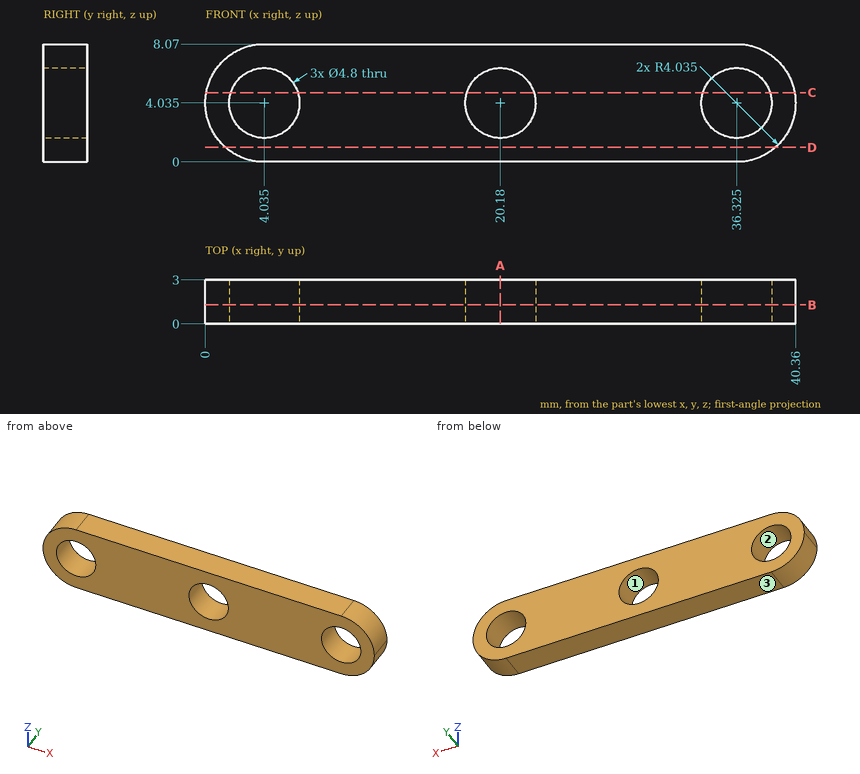
Verification items for this drawing (mm, ordinates from the low corner). Give positions to 0.01 mm unless a question says otherwise; leave off trailing zeros. Write each loop counter-clockwise with the first axis right and the second up, starting at its lowest first coordinate (ties: lowest second). Pieces come first, ordered by that corner, then holes. Notation, with made-up numbers: (66.5, 59) -> (70.5, 59) arc R16 ccw to (70.5, 77) -> close; hole circle Ø6 at (-2, 1). An arc over 180 degrees is marked (long way). Use one line per item in the form item = value.
Item 1: Depth check by flat-ended pin: pin 1 Ø1.5 at (x, z) = (24, 2.5) entering from -Y. Enter the tip coordinate at first touch or a pass-through.
Results list:
pin_1 = 0
Item 2: Scan lines: line 1 (X direction, y = 1.3, z = 4.25); line 2 (X direction, y = 1.5, z = 4.75); line 3 (Z direction, x = 18, y = 1.55). Record each from-to range of solid material in increasing order.
Results list:
line_1 = 0.01 to 1.64, 6.43 to 17.79, 22.57 to 33.93, 38.72 to 40.35
line_2 = 0.06 to 1.74, 6.33 to 17.89, 22.47 to 34.03, 38.62 to 40.3
line_3 = 0 to 3.03, 5.04 to 8.07
Item 3: Sectioned sample at D-D on z = 1. Enter the section's corners in (x, y).
Results list:
outline = (1.38, 0) -> (38.98, 0) -> (38.98, 3) -> (1.38, 3) -> close
Item 4: Mould release check, pull along X, two halves, no side actions. Record for the marked faces 1, 2 and 3: released by +X, released by -X, zero draft, split by the parting line, or undercut.
Results list:
face_1 = undercut
face_2 = undercut
face_3 = zero draft
Item 5: Sectioned sample at B-B on y = 1.3. Enter the section's corners in (x, z) (3 decimals).
Results list:
outline = (4.035, 0) -> (36.325, 0) arc R4.035 ccw to (36.325, 8.07) -> (4.035, 8.07) arc R4.035 ccw to start; hole circle Ø4.8 at (4.035, 4.035); hole circle Ø4.8 at (20.18, 4.035); hole circle Ø4.8 at (36.325, 4.035)
Item 6: Sectioned sample at A-A on x = 20.18. Enter the section's corners in (y, z) (3 decimals), plus the area to 3 significant figures.
Results list:
outline = (0, 0) -> (3, 0) -> (3, 1.635) -> (0, 1.635) -> close; (0, 6.435) -> (3, 6.435) -> (3, 8.07) -> (0, 8.07) -> close
area = 9.81 mm2
Item 7: Sectioned sample at C-C on z = 4.75. Enter the section's corners in (x, y).
Results list:
outline = (0.06, 0) -> (1.74, 0) -> (1.74, 3) -> (0.06, 3) -> close; (6.33, 0) -> (17.89, 0) -> (17.89, 3) -> (6.33, 3) -> close; (22.47, 0) -> (34.03, 0) -> (34.03, 3) -> (22.47, 3) -> close; (38.62, 0) -> (40.3, 0) -> (40.3, 3) -> (38.62, 3) -> close
